Source: CAD feature listing. Evaluate the final solid. Frame: model axes, mm. Round coordinates to 2 decimals unless told otherwise and drop trailing zeros. Loops run counter-clockwise (first coordinate to the right, second up) from the corner with the lowest first, then second, coordinate; pieces in that order, holes last. Notation, with made-up numbers: M -36,27 L -21,27 A18 cw -21,37 Z; hole C -2,50.5 d8. An arc over 180 degrees is marked long. Answer as a JSON object with one key per item and string values.
from build123d import *

# Parameters (mm, degrees)
SKETCH1_W           = 150
SKETCH1_H           = 40
SKETCH1_R           = 11
BOSS_EXTRUDE1_DEPTH = 3


with BuildPart() as part:
    # Sketch1 → Boss-Extrude1 (new, symmetric)
    with BuildSketch(Plane(origin=(0, 0, 0), x_dir=(0, 0, -1), z_dir=(1, 0, 0))):
        Rectangle(SKETCH1_W, SKETCH1_H)
        with Locations((52.481264033, 0)):
            Circle(SKETCH1_R, mode=Mode.SUBTRACT)
    extrude(amount=BOSS_EXTRUDE1_DEPTH, both=True)


solid = part.part
Item 1: Line query: probe 1 along Z at (x, y) = (2.4, 5.5); probe 2 along Z at (x, y) = (-2.6, 6). Output: solid intervals per line, ascending. Write a range as from..to.
Answer sheet:
{"probe 1": "z = -75..-62.01, -42.95..75", "probe 2": "z = -75..-61.7, -43.26..75"}
Item 2: Contact query for a flat-ended pin moving along its axis: pin 1 Ø20 at (y, z) = (0, -52.48) entering from +X. Output: stop coordinate, or through.
Answer sheet:
{"pin 1": "passes through"}
Item 3: Section B-B on z = -48.5. Return the cut outline in (x, y).
Answer sheet:
{"outline": "M -3,-20 L 3,-20 L 3,-10.25 L -3,-10.25 Z; M -3,10.25 L 3,10.25 L 3,20 L -3,20 Z"}
Item 4: Section A-A on y = 0. Return the cut outline in (x, z), then the cut area to 3 significant figures.
Answer sheet:
{"outline": "M -3,-75 L 3,-75 L 3,-63.48 L -3,-63.48 Z; M -3,-41.48 L 3,-41.48 L 3,75 L -3,75 Z", "area": "768 mm²"}
Item 5: Section C-C on x = -0.35. Return the cut outline in (y, z), then the cut area to 3 significant figures.
Answer sheet:
{"outline": "M -20,-75 L 20,-75 L 20,75 L -20,75 Z; hole C 0,-52.48 d22", "area": "5,620 mm²"}
